from build123d import *

# Parameters (mm, degrees)
SKETCH1_R           = 1.5
BOSS_EXTRUDE1_DEPTH = 1.6
BOSS_EXTRUDE2_START = -11
BOSS_EXTRUDE2_DEPTH = 6
SKETCH5_W           = 10
SKETCH5_H           = 6
BOSS_EXTRUDE3_DEPTH = 7


with BuildPart() as part:
    # Sketch1 → Boss-Extrude1 (new body)
    with BuildSketch(Plane(origin=(0, 0, 0), x_dir=(1, 0, 0), z_dir=(0, 1, 0))):
        with BuildLine():
            Line((-5.5, 28), (-3.5, 28))
            ThreePointArc((-3.5, 28), (0, 31.5), (3.5, 28))
            Line((3.5, 28), (5.5, 28))
            Line((5.5, 28), (5.5, 0))
            Line((5.5, 0), (3.5, 0))
            ThreePointArc((3.5, 0), (0, -3.5), (-3.5, 0))
            Line((-3.5, 0), (-5.5, 0))
            Line((-5.5, 0), (-5.5, 28))
        make_face()
        Circle(SKETCH1_R, mode=Mode.SUBTRACT)
        with Locations((0, 28)):
            Circle(SKETCH1_R, mode=Mode.SUBTRACT)
    extrude(amount=BOSS_EXTRUDE1_DEPTH)

    # Sketch3 → Boss-Extrude2 (add)
    with BuildSketch(Plane(origin=(5.5, 0, 0), x_dir=(0, 0, -1), z_dir=(1, 0, 0)).offset(BOSS_EXTRUDE2_START)):
        Polygon((4, 1.6), (4, 11.6), (8, 11.6), (8, 3.6), (13, 3.6), (13, 11.6), (17, 11.6), (17, 1.6), align=None)
    extrude(amount=BOSS_EXTRUDE2_DEPTH)

    # Sketch5 → Boss-Extrude3 (add)
    with BuildSketch(Plane.XZ):
        with Locations((0, -21.8)):
            Rectangle(SKETCH5_W, SKETCH5_H)
    extrude(amount=BOSS_EXTRUDE3_DEPTH)


solid = part.part
Source: CAD feature listing. Evaluate the final solid. Frame: model axes, mm. A direction names the side the tool comes from. Give positions to 0.01 mm unless a question says otherwise; leave off trailing zeros. Write each loop counter-clockwise with the first axis right and the second up, starting at its lowest first coordinate (ties: lowest second). Pieces come first, ordered by that corner, then holes. Notation, with made-up numbers: M 61,-6.5 L 75,-6.5 A20 cw 75,4.5 Z; hole C 42,22.25 d2. An arc over 180 degrees is marked long. Answer as a JSON object with one key per item and string values.
Q1. Contact query for flat-ended pins moving along their axis: P1, Ø3, axis at y = -3.5, z = -20.5, coming from the +X side; P2, Ø4, axis at x = 0, z = -28, coming from the +Y side; P3, Ø1.3, axis at x = 5, y = 1, coming from the +Z side; P4, Ø2, axis at y = -2.5, z = -11, coming from the +X side. Output: stop coordinate, or through.
Geometry check:
{"P1": "stops at x = 5", "P2": "stops at y = 1.6", "P3": "stops at z = 0", "P4": "passes through"}
Q2. Ray query, line 1 along Z through (x, y) = (0, 0.4); line 2 along Z through (x, y) = (-4, 5.75); line 3 along Z through (x, y) = (-2, -4.25). Return the intervals inside material, ascending.
Geometry check:
{"line 1": "z = -31.5 to -29.5, -26.5 to -1.5, 1.5 to 3.5", "line 2": "z = -17 to -13, -8 to -4", "line 3": "z = -24.8 to -18.8"}
Q3. Cut plane B-B, the plane y = 1. Return the cut outline in (x, z), then the cut area to 3 significant figures.
Geometry check:
{"outline": "M -5.5,-28 L -3.5,-28 A3.5 ccw 3.5,-28 L 5.5,-28 L 5.5,0 L 3.5,0 A3.5 ccw -3.5,0 L -5.5,0 Z; hole C 0,-28 d3; hole C 0,0 d3", "area": "332 mm^2"}
Q4. Cut plane D-D, the plane z = -20.5. Return the cut outline in (x, y), then the cut area to 3 significant figures.
Geometry check:
{"outline": "M -5.5,0 L -5,0 L -5,-7 L 5,-7 L 5,0 L 5.5,0 L 5.5,1.6 L -5.5,1.6 Z", "area": "87.6 mm^2"}
Q5. Cut plane A-A, the plane x = 0. Return the cut outline in (y, z).
Geometry check:
{"outline": "M -7,-24.8 L 0,-24.8 L 0,-26.5 L 1.6,-26.5 L 1.6,-17 L 11.6,-17 L 11.6,-13 L 3.6,-13 L 3.6,-8 L 11.6,-8 L 11.6,-4 L 1.6,-4 L 1.6,-1.5 L 0,-1.5 L 0,-18.8 L -7,-18.8 Z; M 0,-31.5 L 1.6,-31.5 L 1.6,-29.5 L 0,-29.5 Z; M 0,1.5 L 1.6,1.5 L 1.6,3.5 L 0,3.5 Z"}
Q6. Access query for faces 1 (the face through (-3, 8, -13)), 2 (the face through (-4, 1, 0)), 3 (the face through (-3, 7, -17)). Directions: +Z, -Z, +X, -X, +Y, -Y. A direction counts if a zero-diameter tool reaches every point of the face in a straight line with its end or side. Return the directions, or none.
Geometry check:
{"face 1": "+X, -X, +Y", "face 2": "+Z, -X, +Y, -Y", "face 3": "-Z, +X, -X, +Y"}
Q7. Mould query, pull axis X, two halves, no side actions, for faces 4 (the face through (0, -7, -22)), 5 (the face through (0.1, 0.8, 3.5)), 6 (the face through (-1.5, 0.79, -0.07)). Classes: +X half, -X half, draft (parallel to the pull), parting line (faces both ways), or undercut.
Geometry check:
{"face 4": "draft", "face 5": "parting line", "face 6": "undercut"}
Q8. Cut plane C-C, the plane y = 9.5. Return the cut outline in (x, z).
Geometry check:
{"outline": "M -5.5,-17 L 0.5,-17 L 0.5,-13 L -5.5,-13 Z; M -5.5,-8 L 0.5,-8 L 0.5,-4 L -5.5,-4 Z"}
